Verification items for the finished model (mm, model axes). A direction names the side the tool comes from. Round coordinates to 2 decimals unless told otherwise and drop trailing zeros. Order: outer loops, then holes, each group sorted by start corner. A loop starts at its lowest first (then second) coordinate and runs counter-clockwise, first axis right, second up. Notation, with made-up numbers: (15, -33) -> (27, -33) arc R23 cw to (27, -16) -> close; hole circle Ø2 at (-9.5, 72.25). An arc over 180 degrees is marked (long way). Put each result on its own line as item: value.
from build123d import *

# Parameters (mm, degrees)
AL_L_ANGLE_ROUNDED_ENDS_L2X1_5X0_125_1_DEPTH = 1016
CUT_EXTRUDE1_DEPTH                           = 512.9533670169578
SKETCH14_R                                   = 4.349749999999978
CUT_EXTRUDE2_DEPTH                           = 512.9533671261084


with BuildPart() as part:
    # Sketch12 → Al l angle (rounded ends) L2X1.5X0.125(1) (new body)
    with BuildSketch(Plane.YZ.offset(-508)):
        with BuildLine():
            Line((0, 0), (-6.94e-15, 50.79999999999999))
            Line((-6.94e-15, 50.79999999999999), (0.00507999999999065, 50.79999999999999))
            ThreePointArc((0.00507999999999065, 50.79999999999999), (2.24655192781885, 49.87155192781885), (3.174999999999991, 47.63007999999999))
            Line((3.174999999999991, 47.63007999999999), (3.1749999999999825, 7.950199999999994))
            ThreePointArc((3.1749999999999825, 7.950199999999994), (4.573623698477981, 4.573623698477992), (7.950199999999982, 3.1749999999999945))
            Line((7.950199999999982, 3.1749999999999945), (34.93008, 3.174999999999994))
            ThreePointArc((34.93008, 3.174999999999994), (37.171551927818854, 2.246551927818857), (38.099999999999994, 0.00507999999999845))
            Line((38.099999999999994, 0.00507999999999845), (38.099999999999994, -1.56e-15))
            Line((38.099999999999994, -1.56e-15), (0, 0))
        make_face()
    extrude(amount=AL_L_ANGLE_ROUNDED_ENDS_L2X1_5X0_125_1_DEPTH)

    # Sketch13 → Cut-Extrude1 (cut, through all)
    with BuildSketch(Plane.XZ):
        with BuildLine():
            Line((-508, 50.79999999999999), (-508, 25.399999999999984))
            ThreePointArc((-508, 25.399999999999984), (-500.5605122421383, 43.3605122421383), (-482.6, 50.79999999999999))
            Line((-482.6, 50.79999999999999), (-508, 50.79999999999999))
        make_face()
        with BuildLine():
            Line((508, 50.79999999999999), (508, 25.399999999999984))
            ThreePointArc((508, 25.399999999999984), (500.5605122421383, 43.3605122421383), (482.6, 50.79999999999999))
            Line((482.6, 50.79999999999999), (508, 50.79999999999999))
        make_face()
    extrude(amount=-CUT_EXTRUDE1_DEPTH, mode=Mode.SUBTRACT)

    # Sketch14 → Cut-Extrude2 (cut, through all)
    with BuildSketch(Plane(origin=(0, 0, 0), x_dir=(-1, 0, 0), z_dir=(0, -4e-17, -1))):
        with Locations(Location((457.20000000000005, 20.000000000006384, 0), (0, 0, 90))):
            Circle(SKETCH14_R)
        with Locations(Location((152.40000000000003, 20.000000000004256, 0), (0, 0, 90))):
            Circle(SKETCH14_R)
        with Locations(Location((-152.39999999999998, 20.000000000002128, 0), (0, 0, 90))):
            Circle(SKETCH14_R)
        with Locations(Location((-457.20000000000005, 20, 0), (0, 0, 90))):
            Circle(SKETCH14_R)
    extrude(amount=-CUT_EXTRUDE2_DEPTH, mode=Mode.SUBTRACT)


solid = part.part
Item 1: Section check B-B on z = 17.5. Record the boundary of the cut face in (x, y) (3 decimals).
Check sheet entries:
outline: (-508, 0) -> (508, 0) -> (508, 3.175) -> (-508, 3.175) -> close
Item 2: Tool access check on faces 4 (the flat face through (-7, 3.175, 28)), 5 (the cylindrical face through (500.76, 1.57, 43.16)). Record the directions out of +Z, -Z, +X, -X, +Y, -Y that give a thin tool (end or side, any length) a straight path to the whole face; none if there is none.
Check sheet entries:
face 4: +Z, +X, -X, +Y
face 5: +Z, +X, +Y, -Y
Item 3: Section check A-A on x = -132. Record the boundary of the cut face in (y, z) (3 decimals), then the cut area to 3 significant figures.
Check sheet entries:
outline: (0, 0) -> (38.1, 0) -> (38.1, 0.005) arc R3.17 ccw to (34.93, 3.175) -> (7.95, 3.175) arc R4.775 cw to (3.175, 7.95) -> (3.175, 47.63) arc R3.17 ccw to (0.005, 50.8) -> (0, 50.8) -> close
area: 273 mm^2
Item 4: Material ranges on L1, parallel to X at y = 20, z = 1.1; L2, parallel to Y at x = 152.4, z = 0.7; L3, parallel to Z at x = -135.5, y = 26.5 (3 decimals), recorded low to high. Write a range as [from, to].
Check sheet entries:
L1: x = [-508, -461.55], [-452.85, -156.75], [-148.05, 148.05], [156.75, 452.85], [461.55, 508]
L2: y = [0, 15.65], [24.35, 38.02]
L3: z = [0, 3.175]
Item 5: Gauge pin test, flat ends, axial feed: pin 1 Ø6 at (y, z) = (5, 18) entering from -X; pin 2 Ø10 at (x, y) = (457.2, 20) entering from +Z (3 decimals); pin 3 Ø4 at (x, z) = (372, 30.5) entering from +Y (3 decimals). Record the tip position at first contact, or that the pin passes through.
Check sheet entries:
pin 1: stops at x = -508
pin 2: stops at z = 3.175
pin 3: stops at y = 3.175
Item 6: Release check for a two-part mould opening along Z. For faces 1 (the flat face through (-7, 21, 3.175)), 2 (the flat face through (-7, 19, 0)), 3 (the flat face through (-7, 0, 25)) record: +Z half, -Z half, draft (parallel to the pull), parting line (faces both ways), or undercut.
Check sheet entries:
face 1: +Z half
face 2: -Z half
face 3: draft
